from build123d import *

# Parameters (mm, degrees)
F0_W     = 50
F0_H     = 45
F1_DEPTH = 6
F3_D     = 6.6
F4_R     = 2


with BuildPart() as f1:
    # F0 (on Front) → F1 (new body)
    with BuildSketch(Plane.XZ):
        with Locations((25, 22.5)):
            Rectangle(F0_W, F0_H)
    extrude(amount=F1_DEPTH)

    # F3 (through all)
    with Locations(Plane.XZ.offset(6)):
        with Locations((10, 39), (25, 35), (40, 39)):
            Hole(F3_D / 2)

    # F4
    f4_edges = [f1.edges().sort_by_distance(p)[0] for p in [
        (50, -3, 0),
        (0, -3, 0),
    ]]
    fillet(f4_edges, radius=F4_R)


solid = f1.part
Could you check a few things on this model? Use its own coordinates, in mm. Give positions to 0.01 mm unless a question says otherwise; leave off trailing zeros. Order: outer loops, then holes, each group sorted by start corner. A loop starts at its lowest first (then second) coordinate and runs counter-clockwise, first axis right, second up. Notation, with made-up numbers: M 65.5,-10 L 87.5,-10 A24 cw 87.5,9 Z; hole C -37,0.5 d7. An arc over 180 degrees is marked long. One line per question, with ' | ' between items.
1. I want a section at C-C (y = -3.55). List the corners of the cut face in (x, z) for me, and give its area (3 significant figures).
Results:
outline: M 0,2 A2 ccw 2,0 L 48,0 A2 ccw 50,2 L 50,45 L 0,45 Z; hole C 10,39 d6.6; hole C 25,35 d6.6; hole C 40,39 d6.6 | area: 2,150 mm²
2. I want a section at D-D (x = 22.5). List the corners of the cut face in (y, z) for me.
Results:
outline: M -6,0 L 0,0 L 0,32.85 L -6,32.85 Z; M -6,37.15 L 0,37.15 L 0,45 L -6,45 Z
3. I'm going to push a flat-ended pin straight in: pin 1 (5.5 mm diameter, centred on x = 25, z = 35, fed in from +Y). Where does the tip first touch, or does it pass through?
Results:
pin 1: through
4. If I drill on line 1 (X direction, y = -1.5, z = 36); line 2 (X direction, y = -5.2, z = 37); line 3 (X direction, y = -4, z = 42), over which ranges is the centre line in solid material (lowest first)?
Results:
line 1: 0 to 8.63, 11.37 to 21.86, 28.14 to 38.63, 41.37 to 50 | line 2: 0 to 7.38, 12.62 to 22.38, 27.62 to 37.38, 42.62 to 50 | line 3: 0 to 8.63, 11.37 to 38.63, 41.37 to 50
5. I want a section at B-B (x = 40). List the corners of the cut face in (y, z) for me, and give its area (3 significant figures).
Results:
outline: M -6,0 L 0,0 L 0,35.7 L -6,35.7 Z; M -6,42.3 L 0,42.3 L 0,45 L -6,45 Z | area: 230 mm²
6. I want a section at A-A (z = 39). List the corners of the cut face in (x, y) for me.
Results:
outline: M 0,-6 L 6.7,-6 L 6.7,0 L 0,0 Z; M 13.3,-6 L 36.7,-6 L 36.7,0 L 13.3,0 Z; M 43.3,-6 L 50,-6 L 50,0 L 43.3,0 Z
